from build123d import *

# Parameters (mm, degrees)
DODANIE_WYCI_GNI_CIE1_DEPTH = 8


with BuildPart() as part:
    # Szkic1 → Dodanie-wyciągnięcie1 (new body)
    with BuildSketch(Plane(origin=(0, 0, 0), x_dir=(1, 0, 0), z_dir=(0, 1, 0))):
        with BuildLine():
            Line((0, 0), (30, 0))
            Line((30, 0), (30, 8.5))
            Line((30, 8.5), (28.5, 8.5))
            ThreePointArc((28.5, 8.5), (27, 10), (28.5, 11.5))
            Line((28.5, 11.5), (30, 11.5))
            Line((30, 11.5), (30, 20))
            Line((30, 20), (0, 20))
            Line((0, 20), (0, 11.5))
            Line((0, 11.5), (1.5, 11.5))
            ThreePointArc((1.5, 11.5), (3, 10), (1.5, 8.5))
            Line((1.5, 8.5), (0, 8.5))
            Line((0, 8.5), (0, 0))
        make_face()
    extrude(amount=DODANIE_WYCI_GNI_CIE1_DEPTH)


solid = part.part
Part model, mm, in its own coordinate system. A direction names the side the tool comes from. Coordinates: 2 decimals unless noted, no trailing zeros. Order: outer loops, then holes, each group sorted by start corner. A loop starts at its lowest first (then second) coordinate and runs counter-clockwise, first axis right, second up. Notation, with made-up numbers: M -8,69.25 L 17,69.25 A10 ccw 17,84.25 Z; hole C 24,-31 d3. An arc over 180 degrees is marked long. Use a Markdown table: item, result.
(1) Tool access for faces 5 (the flat face through (1, 4, -8.5)), 6 (the flat face through (29, 4, -11.5)), 7 (the flat face through (30, 4, -4)): list every direction of +Z, -Z, +X, -X, +Y, -Y with a clear straight run to the whole face (end or side of a thin tool).
A:
| item | result |
|---|---|
| face 5 | -X, +Y, -Y |
| face 6 | +X, +Y, -Y |
| face 7 | +Z, -Z, +X, +Y, -Y |
(2) Flat gauge pin, fed straight in: pin 1 (5 mm diameter, centred on x = 20.5, z = -9, fed in from -Y). Where does the tip first touch, or does it go through?
A:
| item | result |
|---|---|
| pin 1 | stops at y = 0 |
(3) Pull direction Z, two halves, no side cores. Call faces 1 (the flat face through (15, 4, 0)), 2 (the flat face through (0, 4, -16)), 3 (the flat face through (15, 4, -20)), 4 (the cylindrical face through (27, 4, -10)): released by +Z, released by -Z, zero draft, split by the parting line, or undercut.
A:
| item | result |
|---|---|
| face 1 | released by +Z |
| face 2 | zero draft |
| face 3 | released by -Z |
| face 4 | undercut |
(4) Cut at A-A on y = 7.25. Write the cut outline in (x, z).
A:
| item | result |
|---|---|
| outline | M 0,-20 L 30,-20 L 30,-11.5 L 28.5,-11.5 A1.5 cw 28.5,-8.5 L 30,-8.5 L 30,0 L 0,0 L 0,-8.5 L 1.5,-8.5 A1.5 cw 1.5,-11.5 L 0,-11.5 Z |
(5) Probe L1, parallel to Z at x = 2.75, y = 6.25; L2, parallel to X at y = 1, z = -11.25. List the from-to ranges inside material, lowest first.
A:
| item | result |
|---|---|
| L1 | z = -20 to -10.83, -9.17 to 0 |
| L2 | x = 2.33 to 27.67 |
(6) Cut at B-B on z = -10. Write the cut outline in (x, y), then the cut area to 3 significant figures.
A:
| item | result |
|---|---|
| outline | M 3,0 L 27,0 L 27,8 L 3,8 Z |
| area | 192 mm^2 |
